from build123d import *

# Parameters (mm, degrees)
SKETCH1_R                   = 1.2
BOSS_EXTRUDE1_DEPTH         = 1.4
SKETCH2_R                   = 2.25
CUT_EXTRUDE1_DEPTH          = 1.1
CUT_EXTRUDE1_DRAFT          = -45
SKETCH3_W                   = 12
SKETCH3_H                   = 1.5
BOSS_EXTRUDE2_DEPTH         = 3.5
CIRPATTERN1_COUNT           = 2
CIRPATTERN1_ANGLE           = 90
CIRPATTERN1_COPY_1_SKETCH_R = 2.25
CIRPATTERN1_COPY_1_DEPTH    = 1.1
CIRPATTERN1_COPY_1_DRAFT    = -45
CIRPATTERN2_OUTLINE_R       = 2.25
CIRPATTERN2_OUTLINE_R_2     = 1.2
CIRPATTERN2_DEPTH           = 1.4
CIRPATTERN2_START           = -2.1
CIRPATTERN2_2_OUTLINE_W     = 12
CIRPATTERN2_2_OUTLINE_H     = 1.5
CIRPATTERN2_2_OUTLINE_W_2   = 1.5
CIRPATTERN2_2_OUTLINE_H_2   = 12
CIRPATTERN2_2_DEPTH         = 2.1
CIRPATTERN3_COPY_1_SKETCH_R = 2.25
CIRPATTERN3_COPY_1_DEPTH    = 1.1
CIRPATTERN3_COPY_1_DRAFT    = -45
CIRPATTERN3_COPY_2_SKETCH_R = 2.25
CIRPATTERN3_COPY_2_DEPTH    = 1.1
CIRPATTERN3_COPY_2_DRAFT    = -45
CIRPATTERN3_COPY_3_SKETCH_R = 2.25
CIRPATTERN3_COPY_3_DEPTH    = 1.1
CIRPATTERN3_COPY_3_DRAFT    = -45
CUT_EXTRUDE2_DEPTH          = 3
CIRPATTERN4_COUNT           = 4
FILLET2_R                   = 0.25
CUT_EXTRUDE3_DEPTH          = 32.183489221
CUT_EXTRUDE3_DEPTH_BACK     = 32.183489221
SKETCH5_W                   = 28
SKETCH5_H                   = 28
SKETCH5_W_2                 = 27.5
SKETCH5_H_2                 = 27.5
FILLET3_R                   = 2
FILLET4_R                   = 1.1
CUT_EXTRUDE4_DEPTH          = 31.830747639
CUT_EXTRUDE4_DEPTH_BACK     = 31.830747639
SKETCH6_W                   = 0.1
SKETCH6_H                   = 2.1
CUT_EXTRUDE5_DEPTH          = 31.830747639
CUT_EXTRUDE5_DEPTH_BACK     = 31.830747639
SKETCH7_W                   = 0.15
SKETCH7_H                   = 2.1


with BuildPart() as part:
    # Sketch1 → Boss-Extrude1 (new body)
    with BuildSketch(Plane(origin=(0, 0, 0), x_dir=(1, 0, 0), z_dir=(0, 1, 0))):
        Polygon((0, 0), (0, 2), (-6, 2), (-6, -6), (2, -6), (2, 0), align=None)
        with Locations(Location((-2, -2, 0), (0, 0, 270))):
            Circle(SKETCH1_R, mode=Mode.SUBTRACT)
    boss_extrude1 = extrude(amount=BOSS_EXTRUDE1_DEPTH)


with BuildPart() as cut_extrude1_tool:
    # Sketch2 → Cut-Extrude1 (with draft: the straight prism first)
    with BuildSketch(Plane(origin=(0, 1.4, 0), x_dir=(1, 0, 0), z_dir=(0, 1, 0))):
        with Locations((-2, -2)):
            Circle(SKETCH2_R)
    extrude(amount=-CUT_EXTRUDE1_DEPTH)
    # Cut-Extrude1: the draft: its side faces are tilted about the plane it starts from
    cut_extrude1_sides = [cut_extrude1_tool.faces().sort_by_distance(p)[0] for p in [
        (-4.25, 0.85, 2),
    ]]
    draft(cut_extrude1_sides, Plane(origin=(0, 1.4, 0), x_dir=(1, 0, 0), z_dir=(0, 1, 0)), CUT_EXTRUDE1_DRAFT)


with BuildPart() as part_1:
    add(part.part)

    # Cut-Extrude1: cut by cut_extrude1_tool
    add(cut_extrude1_tool.part, mode=Mode.SUBTRACT)

    # Sketch3 → Boss-Extrude2 (add)
    with BuildSketch(Plane(origin=(0, 1.4, 0), x_dir=(1, 0, 0), z_dir=(0, 1, 0))):
        with Locations((8, -0.75)):
            Rectangle(SKETCH3_W, SKETCH3_H)
    boss_extrude2 = extrude(amount=-BOSS_EXTRUDE2_DEPTH)

    # CirPattern1: Boss-Extrude1, Boss-Extrude2 ×2 about axis
    cirpattern1_axis = Axis((8, 0, -8), (0, 1, 0))
    add([boss_extrude1.rotate(cirpattern1_axis, i * CIRPATTERN1_ANGLE / (CIRPATTERN1_COUNT - 1)) for i in range(1, CIRPATTERN1_COUNT)])
    add([boss_extrude2.rotate(cirpattern1_axis, i * CIRPATTERN1_ANGLE / (CIRPATTERN1_COUNT - 1)) for i in range(1, CIRPATTERN1_COUNT)])


with BuildPart() as cirpattern1_copy_1_tool:
    # CirPattern1 copy 1 sketch → CirPattern1 copy 1 (with draft: the straight prism first)
    with BuildSketch(Plane(origin=(16, 1.4, 0), x_dir=(0, 0, -1), z_dir=(0, 1, 0))):
        with Locations((-2, -2)):
            Circle(CIRPATTERN1_COPY_1_SKETCH_R)
    extrude(amount=-CIRPATTERN1_COPY_1_DEPTH)
    # CirPattern1 copy 1: the draft: its side faces are tilted about the plane it starts from
    cirpattern1_copy_1_sides = [cirpattern1_copy_1_tool.faces().sort_by_distance(p)[0] for p in [
        (18, 0.85, 4.25),
    ]]
    draft(cirpattern1_copy_1_sides, Plane(origin=(16, 1.4, 0), x_dir=(0, 0, -1), z_dir=(0, 1, 0)), CIRPATTERN1_COPY_1_DRAFT)


with BuildPart() as part_2:
    add(part_1.part)

    # CirPattern1 copy 1: cut by cirpattern1_copy_1_tool
    add(cirpattern1_copy_1_tool.part, mode=Mode.SUBTRACT)

    # CirPattern2: read off the stored shape, not the designer's step
    # CirPattern2 outline → CirPattern2 (add)
    with BuildSketch(Plane(origin=(0, 0, 0), x_dir=(1, 0, 0), z_dir=(0, 1, 0))):
        Polygon((22, -6), (22, 2), (17.5, 2), (17.5, 14), (22, 14), (22, 22), (14, 22), (14, 17.5), (2, 17.5), (2, 16), (16, 16), (16, 0), (0, 0), (0, 14), (-1.5, 14), (-1.5, 2), (-6, 2), (-6, -6), (2, -6), (2, -1.5), (14, -1.5), (14, -6), align=None)
        with Locations((-2, -2)):
            Circle(CIRPATTERN2_OUTLINE_R, mode=Mode.SUBTRACT)
        with Locations((18, -2)):
            Circle(CIRPATTERN2_OUTLINE_R_2, mode=Mode.SUBTRACT)
        with Locations((18, 18)):
            Circle(CIRPATTERN2_OUTLINE_R_2, mode=Mode.SUBTRACT)
    extrude(amount=CIRPATTERN2_DEPTH)

    # CirPattern2 2 outline → CirPattern2 2 (add)
    with BuildSketch(Plane(origin=(0, 0, 0), x_dir=(1, 0, 0), z_dir=(0, 1, 0)).offset(CIRPATTERN2_START)):
        with Locations((8, 16.75)):
            Rectangle(CIRPATTERN2_2_OUTLINE_W, CIRPATTERN2_2_OUTLINE_H)
        with Locations((-0.75, 8)):
            Rectangle(CIRPATTERN2_2_OUTLINE_W_2, CIRPATTERN2_2_OUTLINE_H_2)
    extrude(amount=CIRPATTERN2_2_DEPTH)

    # Mirror1: Boss-Extrude1 across plane
    add(boss_extrude1.mirror(Plane(origin=(0, 0, -8), x_dir=(1, 0, 0), z_dir=(0, 0, -1))))


with BuildPart() as cirpattern3_copy_1_tool:
    # CirPattern3 copy 1 sketch → CirPattern3 copy 1 (with draft: the straight prism first)
    with BuildSketch(Plane(origin=(16, 1.4, 0), x_dir=(0, 0, -1), z_dir=(0, 1, 0))):
        with Locations((-2, -2)):
            Circle(CIRPATTERN3_COPY_1_SKETCH_R)
    extrude(amount=-CIRPATTERN3_COPY_1_DEPTH)
    # CirPattern3 copy 1: the draft: its side faces are tilted about the plane it starts from
    cirpattern3_copy_1_sides = [cirpattern3_copy_1_tool.faces().sort_by_distance(p)[0] for p in [
        (18, 0.85, 4.25),
    ]]
    draft(cirpattern3_copy_1_sides, Plane(origin=(16, 1.4, 0), x_dir=(0, 0, -1), z_dir=(0, 1, 0)), CIRPATTERN3_COPY_1_DRAFT)


with BuildPart() as part_3:
    add(part_2.part)

    # CirPattern3 copy 1: cut by cirpattern3_copy_1_tool
    add(cirpattern3_copy_1_tool.part, mode=Mode.SUBTRACT)


with BuildPart() as cirpattern3_copy_2_tool:
    # CirPattern3 copy 2 sketch → CirPattern3 copy 2 (with draft: the straight prism first)
    with BuildSketch(Plane(origin=(16, 1.4, -16), x_dir=(-1, 0, 0), z_dir=(0, 1, 0))):
        with Locations((-2, -2)):
            Circle(CIRPATTERN3_COPY_2_SKETCH_R)
    extrude(amount=-CIRPATTERN3_COPY_2_DEPTH)
    # CirPattern3 copy 2: the draft: its side faces are tilted about the plane it starts from
    cirpattern3_copy_2_sides = [cirpattern3_copy_2_tool.faces().sort_by_distance(p)[0] for p in [
        (20.25, 0.85, -18),
    ]]
    draft(cirpattern3_copy_2_sides, Plane(origin=(16, 1.4, -16), x_dir=(-1, 0, 0), z_dir=(0, 1, 0)), CIRPATTERN3_COPY_2_DRAFT)


with BuildPart() as part_4:
    add(part_3.part)

    # CirPattern3 copy 2: cut by cirpattern3_copy_2_tool
    add(cirpattern3_copy_2_tool.part, mode=Mode.SUBTRACT)


with BuildPart() as cirpattern3_copy_3_tool:
    # CirPattern3 copy 3 sketch → CirPattern3 copy 3 (with draft: the straight prism first)
    with BuildSketch(Plane(origin=(0, 1.4, -16), x_dir=(0, 0, 1), z_dir=(0, 1, 0))):
        with Locations((-2, -2)):
            Circle(CIRPATTERN3_COPY_3_SKETCH_R)
    extrude(amount=-CIRPATTERN3_COPY_3_DEPTH)
    # CirPattern3 copy 3: the draft: its side faces are tilted about the plane it starts from
    cirpattern3_copy_3_sides = [cirpattern3_copy_3_tool.faces().sort_by_distance(p)[0] for p in [
        (-2, 0.85, -20.25),
    ]]
    draft(cirpattern3_copy_3_sides, Plane(origin=(0, 1.4, -16), x_dir=(0, 0, 1), z_dir=(0, 1, 0)), CIRPATTERN3_COPY_3_DRAFT)


with BuildPart() as part_5:
    add(part_4.part)

    # CirPattern3 copy 3: cut by cirpattern3_copy_3_tool
    add(cirpattern3_copy_3_tool.part, mode=Mode.SUBTRACT)

    # Sketch4 → Cut-Extrude2 (cut)
    with BuildSketch(Plane.XY.offset(1.5)):
        with BuildLine():
            Line((6.5, 1.4), (9.5, 1.4))
            Line((9.5, 1.4), (9.5, 1.2))
            ThreePointArc((9.5, 1.2), (9.412132034, 0.987867966), (9.2, 0.9))
            Line((9.2, 0.9), (6.8, 0.9))
            ThreePointArc((6.8, 0.9), (6.587867966, 0.987867966), (6.5, 1.2))
            Line((6.5, 1.2), (6.5, 1.4))
        make_face()
    cut_extrude2 = extrude(amount=-CUT_EXTRUDE2_DEPTH, mode=Mode.SUBTRACT)

    # CirPattern4: Cut-Extrude2 ×4 about axis
    cirpattern4_axis = Axis((8, 0, -8), (0, 1, 0))
    for i in range(1, CIRPATTERN4_COUNT):
        add(cut_extrude2.rotate(cirpattern4_axis, i * 360 / CIRPATTERN4_COUNT), mode=Mode.SUBTRACT)

    # Fillet2
    fillet2_edges = [part_5.edges().sort_by_distance(p)[0] for p in [
        (6.5, 1.3, 0),
        (9.5, 1.3, 0),
        (9.412132034, 0.987867966, 0),
        (8, 0.9, 0),
        (6.587867966, 0.987867966, 0),
        (6.5, 1.3, 1.5),
        (6.587867966, 0.987867966, 1.5),
        (8, 0.9, 1.5),
        (9.412132034, 0.987867966, 1.5),
        (9.5, 1.3, 1.5),
        (16, 1.3, -6.5),
        (16, 1.3, -9.5),
        (16, 0.987867966, -9.412132034),
        (16, 0.9, -8),
        (16, 0.987867966, -6.587867966),
        (17.5, 1.3, -6.5),
        (17.5, 0.987867966, -6.587867966),
        (17.5, 0.9, -8),
        (17.5, 0.987867966, -9.412132034),
        (17.5, 1.3, -9.5),
        (9.5, 1.3, -16),
        (6.5, 1.3, -16),
        (6.587867966, 0.987867966, -16),
        (8, 0.9, -16),
        (9.412132034, 0.987867966, -16),
        (9.5, 1.3, -17.5),
        (9.412132034, 0.987867966, -17.5),
        (8, 0.9, -17.5),
        (6.587867966, 0.987867966, -17.5),
        (6.5, 1.3, -17.5),
        (0, 1.3, -9.5),
        (0, 1.3, -6.5),
        (0, 0.987867966, -6.587867966),
        (0, 0.9, -8),
        (0, 0.987867966, -9.412132034),
        (-1.5, 1.3, -9.5),
        (-1.5, 0.987867966, -9.412132034),
        (-1.5, 0.9, -8),
        (-1.5, 0.987867966, -6.587867966),
        (-1.5, 1.3, -6.5),
    ]]
    fillet(fillet2_edges, radius=FILLET2_R)

    # Sketch5 → Cut-Extrude3 (cut, two sides: drawn at the far end of the back side and taken through both)
    with BuildSketch(Plane(origin=(0, 0, 0), x_dir=(1, 0, 0), z_dir=(0, 1, 0)).offset(-CUT_EXTRUDE3_DEPTH_BACK)):
        with Locations((8, 8)):
            Rectangle(SKETCH5_W, SKETCH5_H)
        with Locations((8, 8)):
            Rectangle(SKETCH5_W_2, SKETCH5_H_2, mode=Mode.SUBTRACT)
    extrude(amount=CUT_EXTRUDE3_DEPTH + CUT_EXTRUDE3_DEPTH_BACK, mode=Mode.SUBTRACT)

    # Fillet3
    fillet3_edges = [part_5.edges().sort_by_distance(p)[0] for p in [
        (16, 0.7, -16),
        (0, 0.7, 0),
        (0, 0.7, -16),
        (16, 0.7, 0),
    ]]
    fillet(fillet3_edges, radius=FILLET3_R)

    # Fillet4
    fillet4_edges = [part_5.edges().sort_by_distance(p)[0] for p in [
        (17.5, 0.7, -14),
        (14, 0.7, -17.5),
        (-1.5, 0.7, -2),
        (-1.5, 0.7, -14),
        (2, 0.7, -17.5),
        (2, 0.7, 1.5),
        (14, 0.7, 1.5),
        (17.5, 0.7, -2),
    ]]
    fillet(fillet4_edges, radius=FILLET4_R)

    # Sketch6 → Cut-Extrude4 (cut, two sides: drawn at the far end of the back side and taken through both)
    with BuildSketch(Plane.XY.offset(-CUT_EXTRUDE4_DEPTH_BACK)):
        with Locations((13.95, -1.05)):
            Rectangle(SKETCH6_W, SKETCH6_H)
        with Locations((2.05, -1.05)):
            Rectangle(SKETCH6_W, SKETCH6_H)
    extrude(amount=CUT_EXTRUDE4_DEPTH + CUT_EXTRUDE4_DEPTH_BACK, mode=Mode.SUBTRACT)

    # Sketch7 → Cut-Extrude5 (cut, two sides: drawn at the far end of the back side and taken through both)
    with BuildSketch(Plane(origin=(0, 0, 0), x_dir=(0, 0, -1), z_dir=(1, 0, 0)).offset(-CUT_EXTRUDE5_DEPTH_BACK)):
        with Locations((2.075, -1.05)):
            Rectangle(SKETCH7_W, SKETCH7_H)
        with Locations((13.925, -1.05)):
            Rectangle(SKETCH7_W, SKETCH7_H)
    extrude(amount=CUT_EXTRUDE5_DEPTH + CUT_EXTRUDE5_DEPTH_BACK, mode=Mode.SUBTRACT)


solid = part_5.part
Can you work these out from the model? Positions are in its coordinate system, mm. A direction names the side the tool comes from. Round coordinates to 2 decimals unless told otherwise and drop trailing zeros. Write each loop counter-clockwise with the first axis right and the second up, starting at its lowest first coordinate (ties: lowest second). Pieces come first, ordered by that corner, then holes. Notation, with made-up numbers: M 59,-2.75 L 114,-2.75 A9 cw 114,7.25 Z; hole C 48.5,31.25 d9. An arc over 180 degrees is marked long. Use CSV: the item, a comma, the result in double quotes.
(1) Imagine slicing it at C-C (z = -4.5). Write out the boundary of the cut face in (x, y).
Check values:
outline,"M -1.5,-2.1 L 0,-2.1 L 0,1.4 L -1.5,1.4 Z; M 16,-2.1 L 17.5,-2.1 L 17.5,1.4 L 16,1.4 Z"
(2) I need wall thicknesses on line 1 along X through (y, z) = (-0.7, -7.75); line 2 along Z through (x, y) = (8.75, 0.5); line 3 along Z through (x, y) = (-2, 0.15). Which ranges of each line are inside material? Lowest first, please.
Check values:
line 1,"-1.5 to 0, 16 to 17.5"
line 2,"-17.5 to -16, 0 to 1.5"
line 3,"-21.75 to -19.2, -16.8 to -13.82, -2.18 to 0.8, 3.2 to 5.75"
(3) Imagine slicing it at B-B (x = 11.75). Write out the boundary of the cut face in (y, z), plus the area to 3 significant figures.
Check values:
outline,"M -2.1,-17.5 L 1.4,-17.5 L 1.4,-16 L -2.1,-16 Z; M -2.1,0 L 1.4,0 L 1.4,1.5 L -2.1,1.5 Z"
area,"10.5 mm^2"
(4) Imagine slicing it at A-A (y = -0.8). Write out the boundary of the cut face in (x, z).
Check values:
outline,"M -1.5,-13.85 L 0,-13.85 L 0,-2.15 L -1.5,-2.15 Z; M 2.1,-17.5 L 13.9,-17.5 L 13.9,-16 L 2.1,-16 Z; M 2.1,0 L 13.9,0 L 13.9,1.5 L 2.1,1.5 Z; M 16,-13.85 L 17.5,-13.85 L 17.5,-2.15 L 16,-2.15 Z"
(5) We'd pull the mould along Z, two halves only. Please class faces 5 (the flat face through (0.3, 1.4, -16.9)), 6 (the cylindrical face through (17.814, 0.69, -13.669)), 7 (the flat face through (18, 1, -21.75)): +Z half, -Z half, draft (parallel to the pull), parting line (faces both ways), or undercut.
Check values:
face 5,"draft"
face 6,"undercut"
face 7,"-Z half"
(6) On a 3-axis mill with a long thin cutter (end or side, diameter ignored), from which of +Z, -Z, +X, -X, +Y, -Y can I reach the whole of each face in a straight line? I mean faces 1 (the cylindrical face through (2.331, 0.69, 1.814)), 2 (the flat face through (17, -1, -13.85)), 3 (the flat face through (-4, 1, -2)), 4 (the cylindrical face through (15.4, 0.71, -15.43)). Say none if no direction works.
Check values:
face 1,"+Z, +Y, -Y"
face 2,"-Z, +X, -X, -Y"
face 3,"-X, +Y, -Y"
face 4,"+Y, -Y"
(7) I'm going to push flat-ended pins straight in: pin 1 (1.2 mm diameter, centred on x = -1, y = -1, fed in from +Z); pin 2 (1 mm diameter, centred on x = 9.5, y = 0, fed in from -Z); pin 3 (0.8 mm diameter, centred on x = -1, z = -7.5, fed in from +Y); pin 4 (3 mm diameter, centred on x = 3, z = -8, fed in from -Y). Where does each tip first touch, or does it pass through?
Check values:
pin 1,"z = -2.15"
pin 2,"z = -17.5"
pin 3,"y = 0.9"
pin 4,"through"
(8) Imagine slicing it at D-D (z = -18). Write out the boundary of the cut face in (x, y), plus the area to 3 significant figures.
Check values:
outline,"M -5.75,0 L -3.2,0 L -3.2,0.35 L -4.25,1.4 L -5.75,1.4 Z; M -0.8,0 L 2.18,0 L 2.18,1.4 L 0.25,1.4 L -0.8,0.35 Z; M 13.82,0 L 16.8,0 L 16.8,0.35 L 15.75,1.4 L 13.82,1.4 Z; M 19.2,0 L 21.75,0 L 21.75,1.4 L 20.25,1.4 L 19.2,0.35 Z"
area,"13.3 mm^2"
